Here's how the part is built. I have some questions about the finished solid (model axes, mm). Face numbers are marked on the shaded views. A direction names the side the tool comes from. Round coordinates to 2 decimals unless told otherwise and drop trailing zeros. Order: outer loops, then holes, each group sorted by start corner. A loop starts at its lowest first (then second) coordinate and runs counter-clockwise, first axis right, second up. Notation, with made-up numbers: (-26, 73.5) -> (24, 73.5) arc R22 cw to (24, 93.5) -> close; hole circle Ø10 at (34, -9). An arc over 180 degrees is marked (long way). One line per item, written item: value.
Autodesk Inventor part; units mm, degrees
ref_plane "YZ Plane" through (0, 0, 0) normal (1, 0, 0) x (0, 1, 0)
ref_plane "XZ Plane" through (0, 0, 0) normal (0, 1, 0) x (-1, 0, 0)
ref_plane "XY Plane" through (0, 0, 0) normal (0, 0, 1) x (1, 0, 0)
sketch "Sketch1" plane through (0, 0, 0) normal (0, 0, 1) x (1, 0, 0)
  circle A0 centre (0, 0) radius 11
  dimension "d0" = 22
extrude "Extrusion1" add sketch "Sketch1" along normal blind 7
sketch "Sketch2" plane through (0, 0, 7) normal (0, 0, 1) x (1, 0, 0)
  circle A0 centre (0, 0) radius 9
  dimension "d3" = 18
extrude "Extrusion2" add sketch "Sketch2" along normal blind 5
sketch "Sketch3" plane through (0, 0, 12) normal (0, 0, 1) x (1, 0, 0)
  circle A0 centre (0, 0) radius 2.25
  circle A1 centre (6, 0) radius 1.75
  circle A2 centre (-3, 5.1962) radius 1.75
  circle A3 centre (-3, -5.1962) radius 1.75
  dimension "d6" = 4.5
  dimension "d7" = 3.5
  dimension "d8" = 6
  dimension "d11" = 360
extrude "Extrusion3" cut sketch "Sketch3" against normal through all
properties part number "WA005" material "Aluminum 6061"
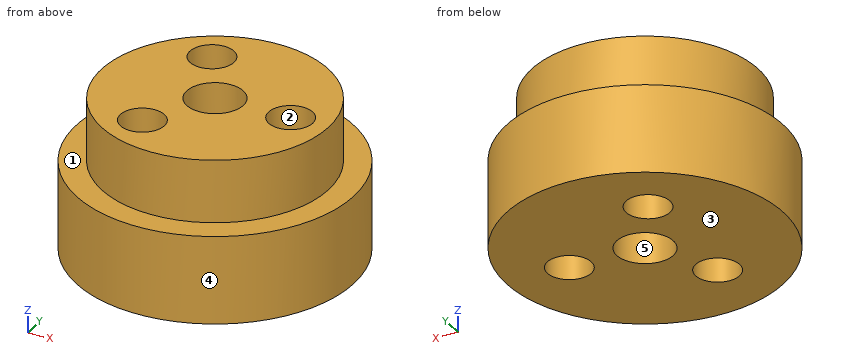
Q1. I want a section at B-B on y = 0. Write out the boundary of the cut face in (x, z).
Answers:
outline: (-11, 0) -> (-2.25, 0) -> (-2.25, 12) -> (-9, 12) -> (-9, 7) -> (-11, 7) -> close; (2.25, 0) -> (4.25, 0) -> (4.25, 12) -> (2.25, 12) -> close; (7.75, 0) -> (11, 0) -> (11, 7) -> (9, 7) -> (9, 12) -> (7.75, 12) -> close
Q2. I want a section at D-D on y = 6.5. Write out the boundary of the cut face in (x, z), then the cut area to 3 significant figures.
Answers:
outline: (-8.87, 0) -> (-4.17, 0) -> (-4.17, 12) -> (-6.22, 12) -> (-6.22, 7) -> (-8.87, 7) -> close; (-1.83, 0) -> (8.87, 0) -> (8.87, 7) -> (6.22, 7) -> (6.22, 12) -> (-1.83, 12) -> close
area: 158 mm2
Q3. I want a section at C-C on x = -3. Write out the boundary of the cut face in (y, z).
Answers:
outline: (-10.58, 0) -> (-6.95, 0) -> (-6.95, 12) -> (-8.49, 12) -> (-8.49, 7) -> (-10.58, 7) -> close; (-3.45, 0) -> (3.45, 0) -> (3.45, 12) -> (-3.45, 12) -> close; (6.95, 0) -> (10.58, 0) -> (10.58, 7) -> (8.49, 7) -> (8.49, 12) -> (6.95, 12) -> close
Q4. For P1, Ø3, axis at y = 4, z = 3, coming from the -X side; P2, Ø1.5, axis at x = -7.5, y = -8, coming from the +Z side; P3, Ø1, axis at y = 5, z = 5, coming from the -X side, each with a flat end and sliding along its axis, tell me the tip position at first contact or that it passes through.
Answers:
P1: x = -10.71
P2: z = 7
P3: x = -10.04
Q5. I need wall thicknesses on line 1 along Y through (x, z) = (-3, 4.25); line 2 along Z through (x, y) = (-0.25, -9.5); line 3 along X through (y, z) = (4.75, 10.75). Which ranges of each line are inside material? Lowest first, please.
Answers:
line 1: -10.58 to -6.95, -3.45 to 3.45, 6.95 to 10.58
line 2: 0 to 7
line 3: -7.64 to -4.69, -1.31 to 7.64
Q6. If we mould it in two halves opening along X, with no side actions, what happens to the marked faces 3, 4 and 5? For each: pulls with the +X half, pulls with the -X half, needs draft (parallel to the pull), parting line crosses it, or undercut.
Answers:
face 3: needs draft
face 4: parting line crosses it
face 5: undercut
Q7. I want a section at A-A on x = 0. Write out the boundary of the cut face in (y, z), then the cut area to 3 significant figures.
Answers:
outline: (-11, 0) -> (-2.25, 0) -> (-2.25, 12) -> (-9, 12) -> (-9, 7) -> (-11, 7) -> close; (2.25, 0) -> (11, 0) -> (11, 7) -> (9, 7) -> (9, 12) -> (2.25, 12) -> close
area: 190 mm2
Q8. Which directions (+Z, -Z, +X, -X, +Y, -Y) give clear straight access to the entire face, cutting with the end or side of a thin tool? Please do the marked faces 1 and 2.
Answers:
face 1: +Z
face 2: +Z, -Z
